from build123d import *

# Parameters (mm, degrees)
SKETCH1_R           = 2.25
BOSS_EXTRUDE1_DEPTH = 6


with BuildPart() as part:
    # Sketch1 → Boss-Extrude1 (new body)
    with BuildSketch(Plane.XY):
        with BuildLine():
            Line((-5, 19), (40, 19))
            ThreePointArc((40, 19), (43.9358142, 15.713699222), (41.404493766, 11.25468329))
            Line((41.404493766, 11.25468329), (1.404493766, -3.74531671))
            ThreePointArc((1.404493766, -3.74531671), (-1.722328125, -3.610205788), (-3.794733192, -1.264911064))
            Line((-3.794733192, -1.264911064), (-8.794733192, 13.735088936))
            ThreePointArc((-8.794733192, 13.735088936), (-8.244968741, 17.338841139), (-5, 19))
        make_face()
        Circle(SKETCH1_R, mode=Mode.SUBTRACT)
        with Locations((-5, 15)):
            Circle(SKETCH1_R, mode=Mode.SUBTRACT)
        with Locations((40, 15)):
            Circle(SKETCH1_R, mode=Mode.SUBTRACT)
    extrude(amount=BOSS_EXTRUDE1_DEPTH)


solid = part.part
For this review, take the finished solid that the model builds, in its own axes (mm). Round coordinates to 2 decimals unless told otherwise and drop trailing zeros. Order: outer loops, then holes, each group sorted by start corner. A loop starts at its lowest first (then second) coordinate and runs counter-clockwise, first axis right, second up. Notation, with made-up numbers: (-21.5, -10) -> (14.5, -10) arc R21 cw to (14.5, 17) -> close; hole circle Ø4 at (29.25, 14). An arc over 180 degrees is marked (long way). Write item = value, one per line. Start each with the question number.
1) The part is to be moulded in two halves that separate along Y. For faces 1 (the face through (-3.962, 13.004, 2.958)), 2 (the face through (21.68, 3.86, 2.96)), 3 (the face through (12, 10, 0)), say which applies: +Y half, -Y half, draft (parallel to the pull), parting line (faces both ways), or undercut.
2) Take a section at B-B on z = 2.15. State the section outline as (x, y) points, plus the area to 3 significant figures.
3) Take a section at C-C on y = 15. State the section outline as (x, z) points, plus the area to 3 significant figures.
4) To check wall thickness, follow line 1 (Y direction, x = 0, z = 4.6); line 2 (Y direction, x = 1, z = 3); line 3 (Y direction, x = 30, z = 1.5). State the ranges of each line that lie inside material, in increasing order. Write a range as from..to.
5) Insertion check: pin 1 (1 mm diameter, centred on x = 23, z = 3, fed in from -Y); pin 2 (2 mm diameter, centred on x = 32.5, y = 10, fed in from -Z); pin 3 (2.5 mm diameter, centred on x = 0, y = 0, fed in from -Z); pin 4 (3 mm diameter, centred on y = 0, z = 3, fed in from -X). Each pin has a flat end and moves straight along its axis. Give the tip position at first contact, or say it passes through.
6) Take a section at D-D on x = 29.5. State the section outline as (y, z) points, plus the area to 3 significant figures.
7) Take a section at A-A on x = 0. State the section outline as (y, z) points.
Verdict:
q1.face_1 = undercut
q1.face_2 = -Y half
q1.face_3 = draft
q2.outline = (-8.79, 13.74) -> (-3.79, -1.26) arc R4 ccw to (1.4, -3.75) -> (41.4, 11.25) arc R4 ccw to (40, 19) -> (-5, 19) arc R4 ccw to start; hole circle Ø4.5 at (-5, 15); hole circle Ø4.5 at (0, 0); hole circle Ø4.5 at (40, 15)
q2.area = 754 mm2
q3.outline = (-9, 0) -> (-7.25, 0) -> (-7.25, 6) -> (-9, 6) -> close; (-2.75, 0) -> (37.75, 0) -> (37.75, 6) -> (-2.75, 6) -> close; (42.25, 0) -> (44, 0) -> (44, 6) -> (42.25, 6) -> close
q3.area = 264 mm2
q4.line_1 = -4..-2.25, 2.25..19
q4.line_2 = -3.87..-2.02, 2.02..19
q4.line_3 = 6.98..19
q5.pin_1 = 4.17
q5.pin_2 = 0
q5.pin_3 = through
q5.pin_4 = -4.72
q6.outline = (6.79, 0) -> (19, 0) -> (19, 6) -> (6.79, 6) -> close
q6.area = 73.3 mm2
q7.outline = (-4, 0) -> (-2.25, 0) -> (-2.25, 6) -> (-4, 6) -> close; (2.25, 0) -> (19, 0) -> (19, 6) -> (2.25, 6) -> close
